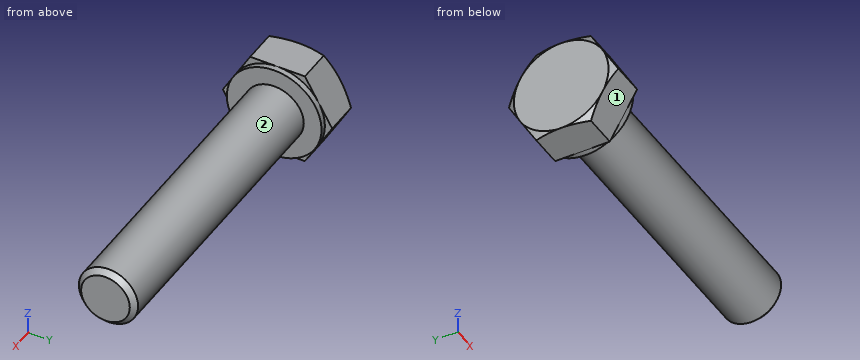
```python
from build123d import *

# Parameters (mm, degrees)
BASEHEAD_DEPTH = 3.65
SKETCH4_W      = 0.5
SKETCH4_H      = 10.618802154


# Read off the part's stored shape, not the designer's step: HeadChamfer
with BuildPart() as part:
    # Sketch1 → BaseHead (new body)
    with BuildSketch(Plane(origin=(0, 0, 0), x_dir=(0, 0, -1), z_dir=(1, 0, 0))):
        Polygon((4, 2.309401077), (4, -2.309401077), (0, -4.618802154), (-4, -2.309401077), (-4, 2.309401077), (0, 4.618802154), align=None)
    extrude(amount=BASEHEAD_DEPTH)

    # HeadChamfer outline → HeadChamfer (revolve, cut)
    with BuildSketch(Plane.YX):
        Polygon((4.618802148, 0.357265587), (3.999999382, -3.57e-07), (4.618802154, -3.57e-07), align=None)
    revolve(axis=Axis((0, 0, 0), (1, 0, 0)), mode=Mode.SUBTRACT)

    # HeadChamfer 2 outline → HeadChamfer 2 (revolve)
    with BuildSketch(Plane.YX):
        Polygon((2.5, 3.65), (2.5, 28.205), (2.055, 28.65), (0, 28.65), (0, 3.65), align=None)
    revolve(axis=Axis((0, 0, 0), (1, 0, 0)))

    # Sketch4 → BearingFace (revolve, cut)
    with BuildSketch(Plane.XY, mode=Mode.PRIVATE) as bearingface_sk:
        with Locations((3.4, 9.309401077)):
            Rectangle(SKETCH4_W, SKETCH4_H)
    revolve(bearingface_sk.sketch.rotate(Axis((0, 0, 0), (1, 0, 0)), 90), axis=Axis((0, 0, 0), (1, 0, 0)), mode=Mode.SUBTRACT)


solid = part.part
```
Geometry: final body of the model. Coordinates: model frame, mm. Face numbers are marked on the shaded views. A direction names the side the tool comes from. Coordinates: 2 decimals unless noted, no trailing zeros. Loops run counter-clockwise (first coordinate to the right, second up) from the corner with the lowest first, then second, coordinate; pieces in that order, holes last. Notation, with made-up numbers: (6, 32.25) -> (56, 32.25) arc R22 cw to (56, 58.25) -> close; hole circle Ø10 at (24.5, 82). An arc over 180 degrees is marked (long way). Use a Markdown table: item, result. Add a question column.
(1) Section query A-A, the plane x = 18.25. Return loops of the section in (y, z).
(2) Access query for the marked faces 1 and 2. Directions: +Z, -Z, +X, -X, +Y, -Y. A direction counts if a zero-diameter tool reaches every point of the face in a straight line with its end or side. Return the directions, or none.
(3) Line query: line 1 along X through (y, z) = (2.5, 1); line 2 along Y through (x, z) = (9.5, 1.5); line 3 along Z through (x, y) = (8, 2). Output: solid intervals per line, ascending.
(4) Pin query (flat end, axial travel): pin 1 Ø1.6 at (y, z) = (1.5, -3) entering from +X; pin 2 Ø1.5 at (x, z) = (4, -2.5) entering from +Y; pin 3 Ø1.5 at (x, y) = (14, -1.5) entering from +Z. Return the tip coordinate at first contact, or that it passes through.
Answer:
| question | item | result |
|---|---|---|
| 1 | outline | circle Ø5 at (0, 0) |
| 2 | face 1 | -Z, +X, -X, -Y |
| 2 | face 2 | +X |
| 3 | line 1 | x = 0 to 3.65 |
| 3 | line 2 | y = -2 to 2 |
| 3 | line 3 | z = -1.5 to 1.5 |
| 4 | pin 1 | stops at x = 3.65 |
| 4 | pin 2 | stops at y = 3.55 |
| 4 | pin 3 | stops at z = 2.38 |
